Verification items for this drawing (mm, ordinates from the low corner). Give positions to 0.01 mm unless a question says otherwise; leave off trailing zeros. Write each loop counter-clockwise with the first axis right and the second up, starting at its lowest first coordinate (ties: lowest second). Pieces come first, ordered by that corner, then holes. Notation, with made-up numbers: M -26,-30.5 L -8,-30.5 A24 ccw -8,-4.5 Z; hole C -8,79.5 d1. An arc over 180 degrees is marked long. Write each question's results on one line, items separated by ' | '.
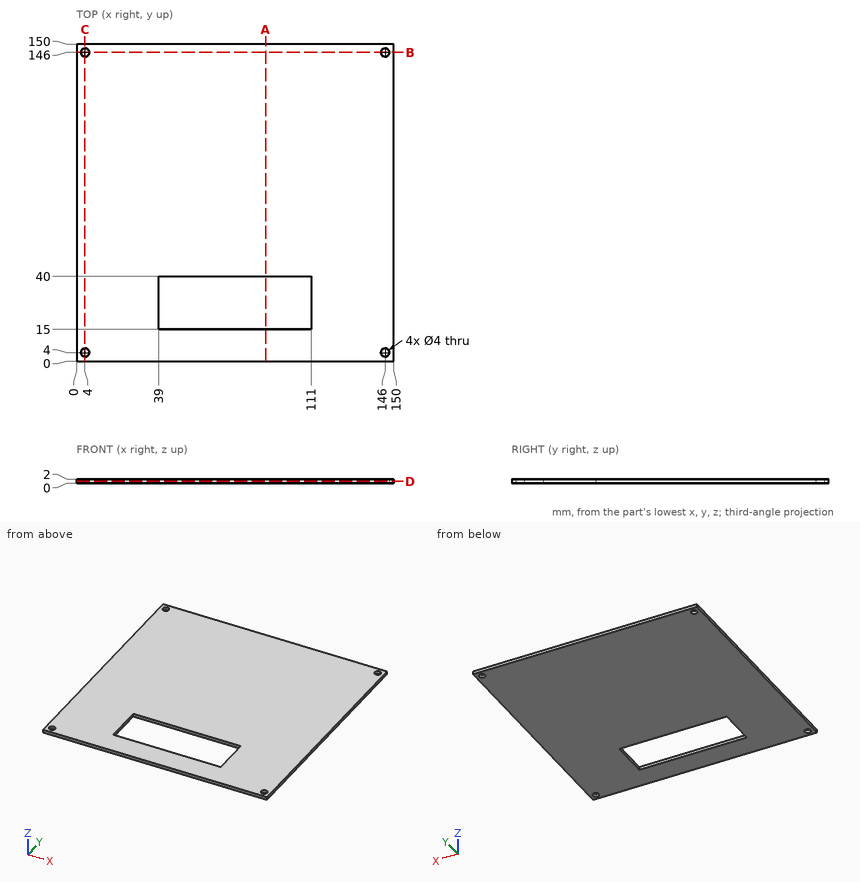
Q1. Depth check by flat-ended pin: P1, Ø5, axis at x = 88.5, y = 109.5, coming from the -Z side; P2, Ø3, axis at x = 4, y = 4, coming from the +Z side. Enter the tip coordinate at first touch or a pass-through.
Answer key:
P1: stops at z = 0 | P2: passes through
Q2. Material ranges on probe 1 along X at (y, z) = (4, 1.1); probe 2 along Y at (x, z) = (88, 0.7), recorded low to high. Write a range as [from, to].
Answer key:
probe 1: x = [0, 2], [6, 144], [148, 150] | probe 2: y = [0, 15], [40, 150]
Q3. Section check A-A (x = 89.5). Enter the section's corners in (y, z).
Answer key:
outline: M 0,0 L 15,0 L 15,2 L 0,2 Z; M 40,0 L 150,0 L 150,2 L 40,2 Z
Q4. Section check B-B (y = 146). Enter the section's corners in (x, z), then the cut area to 3 significant figures.
Answer key:
outline: M 0,0 L 2,0 L 2,2 L 0,2 Z; M 6,0 L 144,0 L 144,2 L 6,2 Z; M 148,0 L 150,0 L 150,2 L 148,2 Z | area: 284 mm2
Q5. Section check D-D (z = 0.9). Enter the section's corners in (x, y).
Answer key:
outline: M 0,0 L 150,0 L 150,150 L 0,150 Z; hole C 4,4 d4; hole C 4,146 d4; hole M 39,15 L 111,15 L 111,40 L 39,40 Z; hole C 146,4 d4; hole C 146,146 d4
